```python
from build123d import *

# Parameters (mm, degrees)
F0_W     = 196
F0_H     = 5
F1_DEPTH = 50
F2_W     = 196
F2_H     = 5
F3_DEPTH = 10
F4_W     = 196
F4_H     = 5
F5_DEPTH = 5
F6_W     = 5.5
F6_H     = 2
F7_DEPTH = 30
F9_DEPTH = 5


with BuildPart() as f1:
    # F0 (on Top) → F1 (new body)
    with BuildSketch(Plane.XY):
        with Locations((98, 2.5)):
            Rectangle(F0_W, F0_H)
    extrude(amount=F1_DEPTH)

    # F2 (on Top) → F3 (join)
    with BuildSketch(Plane.XY):
        with Locations((98, 7.5)):
            Rectangle(F2_W, F2_H)
    extrude(amount=F3_DEPTH)

    # F4 (on Top) → F5 (join)
    with BuildSketch(Plane.XY):
        with Locations((98, 12.5)):
            Rectangle(F4_W, F4_H)
    extrude(amount=F5_DEPTH)

    # F6 (on Top) → F7 (join)
    with BuildSketch(Plane.XY):
        Polygon((0, 18), (0, 15), (4.5, 15), (4.5, 17), (4.5, 18), align=None)
        with Locations((7.25, 16)):
            Rectangle(F6_W, F6_H)
        Polygon((10, 17), (10, 15), (57, 15), (57, 20), (10, 20), align=None)
        Polygon((191.5, 15), (196, 15), (196, 18), (191.5, 18), (191.5, 17), align=None)
        with Locations((188.75, 16)):
            Rectangle(F6_W, F6_H)
        Polygon((139, 15), (186, 15), (186, 17), (186, 20), (139, 20), align=None)
    extrude(amount=F7_DEPTH)

    # F8 (on face) → F9 (join)
    with BuildSketch(Plane(origin=(0, 15, 0), x_dir=(-1, 0, 0), z_dir=(0, 1, 0))):
        Polygon((-139, 0), (-57, 0), (-57, 14), (-67, 14), (-129, 14), (-139, 14), align=None)
        Polygon((-67, 14), (-57, 14), (-57, 30), align=None)
        Polygon((-139, 30), (-139, 14), (-129, 14), align=None)
    extrude(amount=F9_DEPTH)


solid = f1.part
```
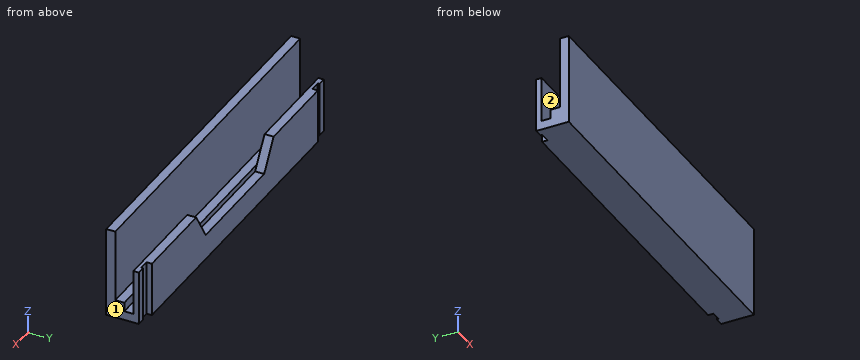
Input: part model. Units: mm. Frame: model coordinates. Face numbers are marked on the shaded views. A direction names the side the tool comes from. Coordinates: 2 decimals unless noted, no trailing zeros. Loops run counter-clockwise (first coordinate to the right, second up) from the corner with the lowest first, then second, coordinate; pieces in that order, holes last. Notation, with made-up numbers: M 8,-12.5 L 66,-12.5 A28 cw 66,21.5 Z; hole C 46.25,-19 d9. An arc over 180 degrees is marked long. Use a Markdown table: item, result. Add a question column.
1) Section D-D, the plane x = 165.5. Return the cut outline in (y, z), plus the area to 3 significant figures.
2) Section C-C, the plane y = 11.75. Return the cut outline in (x, z).
3) Pin query (flat end, axial travel): P1, Ø10, axis at x = 109.5, z = 33, coming from the +Y side; P2, Ø2, axis at x = 193.5, z = 20.5, coming from the +Y side; P3, Ø1.5, axis at x = 84.5, y = 6.5, coming from the +Z side. Return the tip coordinate at first contact, or that it passes through.
4) Section B-B, the plane x = 97. Return the cut outline in (y, z).
5) Set-up query: the marked faces 1 and 2. Return all of +Z, -Z, +X, -X, +Y, -Y with unobstructed straight access to the full face (end or side cutting, diameter ignored); none if empty.
6) Section A-A, the plane z = 19. Return the cut outline in (x, y) (3 decimals).
7) Line query: L1, parallel to Y at x = 137.5, z = 15.5; L2, parallel to X at y = 17.75, z = 3; L3, parallel to Y at x = 116, z = 5.5. Output: solid intervals per line, ascending. Write a range as from..to.
Answer below:
| question | item | result |
|---|---|---|
| 1 | outline | M 0,0 L 20,0 L 20,30 L 15,30 L 15,5 L 10,5 L 10,10 L 5,10 L 5,50 L 0,50 Z |
| 1 | area | 475 mm2 |
| 2 | outline | M 0,0 L 196,0 L 196,5 L 0,5 Z |
| 3 | P1 | y = 5 |
| 3 | P2 | y = 18 |
| 3 | P3 | z = 10 |
| 4 | outline | M 0,0 L 20,0 L 20,14 L 15,14 L 15,5 L 10,5 L 10,10 L 5,10 L 5,50 L 0,50 Z |
| 5 | face 1 | +Z, -Z, +X, +Y, -Y |
| 5 | face 2 | +Z, +X, -X |
| 6 | outline | M 0,0 L 196,0 L 196,5 L 0,5 Z; M 0,15 L 63.875,15 L 63.875,20 L 10,20 L 10,17 L 4.5,17 L 4.5,18 L 0,18 Z; M 132.125,15 L 196,15 L 196,18 L 191.5,18 L 191.5,17 L 186,17 L 186,20 L 132.125,20 Z |
| 7 | L1 | 0..5, 15..20 |
| 7 | L2 | 0..4.5, 10..186, 191.5..196 |
| 7 | L3 | 0..10, 15..20 |
